Design review of the part built by this model. Coordinates are the model's own, in mm. Give positions to 0.01 mm unless a question says otherwise; leave off trailing zeros. Write each loop counter-clockwise with the first axis right and the second up, starting at its lowest first coordinate (ties: lowest second). Pieces come first, ordered by that corner, then holes.
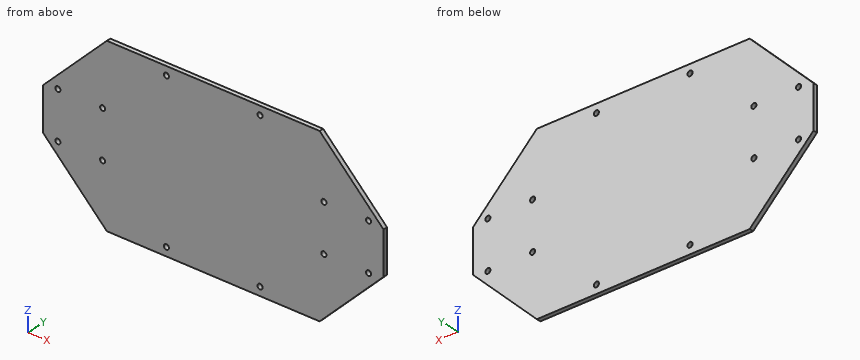
```python
from build123d import *

# Parameters (mm, degrees)
ESQUISSE1_W             = 160
ESQUISSE1_H             = 80
BOSS_EXTRU_1_DEPTH      = 2
ENL_V_MAT_EXTRU_1_DEPTH = 2
D_GAGEMENT_M21_D        = 2.4


with BuildPart() as part:
    # Esquisse1 → Boss.-Extru.1 (new body)
    with BuildSketch(Plane(origin=(0, 0, 0), x_dir=(1, 0, 0), z_dir=(0, 1, 0))):
        with Locations((80, 40)):
            Rectangle(ESQUISSE1_W, ESQUISSE1_H)
    extrude(amount=BOSS_EXTRU_1_DEPTH)

    # Esquisse2 → Enlèv. mat.-Extru.1 (cut)
    with BuildSketch(Plane(origin=(0, 2, 0), x_dir=(1, 0, 0), z_dir=(0, 1, 0))):
        Polygon((0, 30), (30, 0), (0, 0), align=None)
        Polygon((30, 80), (0, 50), (0, 80), align=None)
        Polygon((130, 80), (160, 80), (160, 50), align=None)
        Polygon((160, 30), (130, 0), (160, 0), align=None)
    extrude(amount=-ENL_V_MAT_EXTRU_1_DEPTH, mode=Mode.SUBTRACT)

    # Dégagement M21 (through all)
    with Locations(Plane(origin=(0, 2, 0), x_dir=(1, 0, 0), z_dir=(0, 1, 0))):
        with Locations((7, 51), (7, 29), (28, 29), (28, 51), (58, 76), (58, 4), (132, 29), (153, 29), (153, 51), (132, 51), (101.994988581, 76), (101.994988581, 4)):
            Hole(D_GAGEMENT_M21_D / 2)


solid = part.part
```
(1) Consider section C-C, the plane z = -56. Give the boundary of the cut face in (x, y), then the cut area to 3 significant figures.
Resolved:
outline: (6, 0) - (154, 0) - (154, 2) - (6, 2) - close
area: 296 mm2
(2) To check wall thickness, follow L1, parallel to X at y = 0.8, z = -51; L2, parallel to Z at x = 28, y = 1.15; L3, parallel to Z at x = 153, y = 1.6. State the ranges of each line that lie inside material, in increasing order.
Resolved:
L1: x = 1 to 5.8, 8.2 to 26.8, 29.2 to 130.8, 133.2 to 151.8, 154.2 to 159
L2: z = -78 to -52.2, -49.8 to -30.2, -27.8 to -2
L3: z = -57 to -52.2, -49.8 to -30.2, -27.8 to -23
(3) Consider section A-A, the plane y = 0.3. Give the number of separate pieces and of enclosed holes in the cut face, then the cut area to 3 significant figures.
Resolved:
separate pieces: 1
enclosed holes: 12
area: 10,900 mm2
(4) Consider section B-B, the plane z = -68. Give the boundary of the cut face in (x, y).
Resolved:
outline: (18, 0) - (142, 0) - (142, 2) - (18, 2) - close
